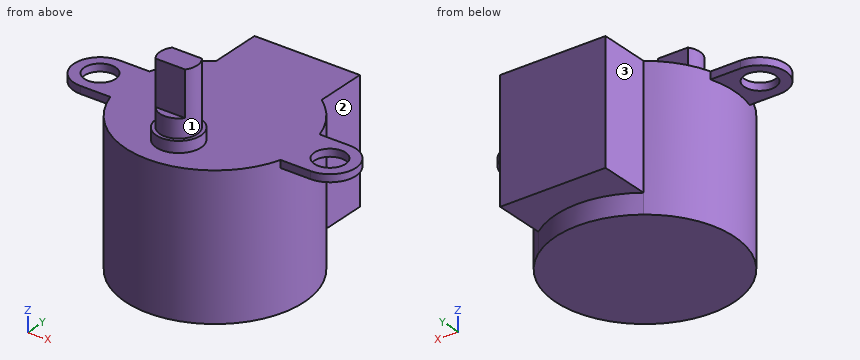
```python
from build123d import *

# Parameters (mm, degrees)
BOSS_EXTRUDE1_DEPTH = 19
CUT_EXTRUDE1_DEPTH  = 2.7
SKETCH3_R           = 2.1
BOSS_EXTRUDE2_DEPTH = 1
SKETCH4_R           = 3
BOSS_EXTRUDE3_DEPTH = 1.5
SKETCH5_R           = 2.5
BOSS_EXTRUDE5_DEPTH = 8.5
CUT_EXTRUDE2_DEPTH  = 6


with BuildPart() as part:
    # Sketch1 → Boss-Extrude1 (new body)
    with BuildSketch(Plane.XY):
        with BuildLine():
            Line((-7.1, 9.674192473), (-7.1, 16.5))
            Line((-7.1, 16.5), (7.1, 16.5))
            Line((7.1, 16.5), (7.1, 9.674192473))
            ThreePointArc((7.1, 9.674192473), (0, -12), (-7.1, 9.674192473))
        make_face()
    extrude(amount=BOSS_EXTRUDE1_DEPTH)

    # Sketch2 → Cut-Extrude1 (cut)
    with BuildSketch(Plane(origin=(0, 0, 0), x_dir=(-1, 0, 0), z_dir=(0, 0, -1))):
        with BuildLine():
            Line((7.1, 16.5), (7.1, 9.674192473))
            ThreePointArc((7.1, 9.674192473), (0, 12), (-7.1, 9.674192473))
            Line((-7.1, 9.674192473), (-7.1, 16.5))
            Line((-7.1, 16.5), (7.1, 16.5))
        make_face()
    extrude(amount=-CUT_EXTRUDE1_DEPTH, mode=Mode.SUBTRACT)

    # Sketch3 → Boss-Extrude2 (add)
    with BuildSketch(Plane.XY.offset(19)):
        with BuildLine():
            Line((-15.5, 3.5), (-11.478240283, 3.5))
            ThreePointArc((-11.478240283, 3.5), (-12, 0), (-11.478240283, -3.5))
            Line((-11.478240283, -3.5), (-15.5, -3.5))
            ThreePointArc((-15.5, -3.5), (-19, 0), (-15.5, 3.5))
        make_face()
        with Locations((-15.5, 0)):
            Circle(SKETCH3_R, mode=Mode.SUBTRACT)
        with BuildLine():
            Line((11.478240283, 3.5), (15.5, 3.5))
            ThreePointArc((15.5, 3.5), (19, 0), (15.5, -3.5))
            Line((15.5, -3.5), (11.478240283, -3.5))
            ThreePointArc((11.478240283, -3.5), (12, 0), (11.478240283, 3.5))
        make_face()
        with Locations((15.5, 0)):
            Circle(SKETCH3_R, mode=Mode.SUBTRACT)
    extrude(amount=-BOSS_EXTRUDE2_DEPTH)

    # Sketch4 → Boss-Extrude3 (add)
    with BuildSketch(Plane.XY.offset(19)):
        with Locations((0, -6.5)):
            Circle(SKETCH4_R)
    extrude(amount=BOSS_EXTRUDE3_DEPTH)

    # Sketch5 → Boss-Extrude5 (add)
    with BuildSketch(Plane.XY.offset(20.5)):
        with Locations((0, -6.5)):
            Circle(SKETCH5_R)
    extrude(amount=BOSS_EXTRUDE5_DEPTH)

    # Sketch7 → Cut-Extrude2 (cut)
    with BuildSketch(Plane.XY.offset(29)):
        with BuildLine():
            Line((-2, -5), (2, -5))
            ThreePointArc((2, -5), (0, -4), (-2, -5))
        make_face()
        with BuildLine():
            Line((-2, -8), (2, -8))
            ThreePointArc((2, -8), (0, -9), (-2, -8))
        make_face()
    extrude(amount=-CUT_EXTRUDE2_DEPTH, mode=Mode.SUBTRACT)


solid = part.part
```
Check sheet for the modelled part. Datum: model origin and axes. Units: mm. Face numbers are marked on the shaded views. A direction names the side the tool comes from. Round coordinates to 2 decimals unless told otherwise and drop trailing zeros. Loops run counter-clockwise (first coordinate to the right, second up) from the corner with the lowest first, then second, coordinate; pieces in that order, holes last. Notation, with made-up numbers: (68.25, -1) - (83.25, -1) arc R25 ccw to (83.25, 18) - close; hole circle Ø3 at (49.25, 82.5). An arc over 180 degrees is marked (long way). Write item = value, one per line. Start each with the question number.
Q1. Depth check by flat-ended pin: P1, Ø3.5, axis at y = 14, z = 12.5, coming from the +X side; P2, Ø0.5, axis at x = -13, z = 18.5, coming from the +Y side; P3, Ø2, axis at x = -17, y = -0.5, coming from the -Z side. Enter the tip coordinate at first touch or a pass-through.
Q2. Access from +Z, -Z, +X, -X, +Y, -Y to the whole of each face (thin tool, end or side, straight path). Record for the marked faces 1, 2 and 3.
Q3. Thickness scan on L1, parallel to Y at x = -15.5, z = 18.45; L2, parallel to Z at x = 10, y = 5.5; L3, parallel to Y at x = 3.5, z = 17.5. Record the ranges inside material, lowest first.
Q4. Section check D-D (y = 11.25). Record the boundary of the cut face in (x, z).
Q5. Section check A-A (x = 0). Record the boundary of the cut face in (y, z), plus the area to 3 significant figures.
Q6. Section check C-C (z = 16.5). Record the boundary of the cut face in (x, y).
Q7. Section check B-B (y = -6.5). Record the boundary of the cut face in (x, z).
Derived:
q1.P1 = 7.1
q1.P2 = 3.5
q1.P3 = 18
q2.face_1 = +Z
q2.face_2 = +Z, -Z, +X, +Y
q2.face_3 = +Z, -Z, -X, +Y
q3.L1 = -3.5 to -2.1, 2.1 to 3.5
q3.L2 = 0 to 19
q3.L3 = -11.48 to 16.5
q4.outline = (-7.1, 2.7) - (-4.18, 2.7) - (-4.18, 0) - (4.18, 0) - (4.18, 2.7) - (7.1, 2.7) - (7.1, 19) - (-7.1, 19) - close
q5.outline = (-12, 0) - (12, 0) - (12, 2.7) - (16.5, 2.7) - (16.5, 19) - (-3.5, 19) - (-3.5, 20.5) - (-4, 20.5) - (-4, 23) - (-5, 23) - (-5, 29) - (-8, 29) - (-8, 23) - (-9, 23) - (-9, 20.5) - (-9.5, 20.5) - (-9.5, 19) - (-12, 19) - close
q5.area = 569 mm^2
q6.outline = (-7.1, 9.67) arc R12 ccw (long way) to (7.1, 9.67) - (7.1, 16.5) - (-7.1, 16.5) - close
q7.outline = (-10.09, 0) - (10.09, 0) - (10.09, 19) - (3, 19) - (3, 20.5) - (2.5, 20.5) - (2.5, 29) - (-2.5, 29) - (-2.5, 20.5) - (-3, 20.5) - (-3, 19) - (-10.09, 19) - close
